Geometry: final body of the model. Coordinates: model frame, mm. A direction names the side the tool comes from. Coordinates: 2 decimals unless noted, no trailing zeros. Order: outer loops, then holes, each group sorted by start corner. A loop starts at its lowest first (then second) coordinate and runs counter-clockwise, first axis right, second up. Notation, with made-up numbers: (31.25, -38.75) -> (37.25, -38.75) arc R27 cw to (37.25, -5.75) -> close; hole circle Ø8 at (81, -34). An arc over 180 degrees is marked (long way). Answer in a Markdown table with one row per item. Add a question column.
1) Section query D-D on y = 61.5. Return the cut outline in (x, z), then the cut area to 3 significant figures.
2) Section query C-C on x = -33.5. Return the cut outline in (y, z), then the cut area to 3 significant figures.
3) Section query B-B on z = 143. Return the cut outline in (x, y), then the cut area to 3 significant figures.
4) Section query A-A on y = 35. Return the cut outline in (x, z).
5) Pull-direction query (Y, two-part tool) for faces 1 (the face through (-32, 85, 78)), 2 (the face through (10.809, 67.931, 77.302)), 3 (the face through (-31, -15, 78)); classes: +Y half, -Y half, draft (parallel to the pull), parting line (faces both ways), or undercut.
6) Contact query for flat-ended pins moving along their axis: P1, Ø8, axis at y = 0, z = 80, coming from the -X side; P2, Ø4, axis at x = -110.5, z = 147, coming from the +Y side; P3, Ø12, axis at x = -30.05, y = 35, coming from the -Z side; P4, Ø1, axis at y = 14.5, z = 31, coming from the -X side. Output: stop coordinate, or through.
7) Set-up query: faces 4 (the face through (10.809, -2.069, 77.302)), 5 (the face through (-55, 36, -34.286)). Return all of +Z, -Z, +X, -X, +Y, -Y with unobstructed straight access to the full face (end or side cutting, diameter ignored); none if empty.
8) Ray query, line 1 (Y direction, x = 4.5, z = 80); line 2 (Z direction, x = 17, y = 0); line 3 (X direction, y = 33, z = 143.5). Return the intervals inside material, ascending. Write a range as from..to.
```python
from build123d import *

# Parameters (mm, degrees)
BOSS_EXTRUDE1_DEPTH    = 160
SCALE1_SCALE           = 1.428571429
F_20_0MM_DOWEL_HOLE1_D = 20
M8_TAPPED_HOLE1_D      = 6.8
M8_TAPPED_HOLE1_DEPTH  = 22.25
M8_TAPPED_HOLE1_TIP    = 2.042926105


with BuildPart() as part:
    # Sketch1 → Boss-Extrude1 (new body)
    with BuildSketch(Plane.XY):
        with BuildLine():
            Line((0, 0), (-75, 0))
            ThreePointArc((-75, 0), (-110, 35), (-75, 70))
            Line((-75, 70), (0, 70))
            Line((0, 70), (0, 0))
        make_face()
    extrude(amount=BOSS_EXTRUDE1_DEPTH)


with BuildPart() as part_1:
    # Scale1: scaled about (-51.542183312, 35, 80)
    add(part.part.scale(SCALE1_SCALE).moved(Location((22.089507134, -15, -34.285714286))))

    # Ø20.0mm Dowel Hole1 (through all)
    with Locations(Plane(origin=(-30.053350009, 35, -34.285714286), x_dir=(-1, 0, 0), z_dir=(0, 0, -1))):
        with Locations((0, 0), (55, 0)):
            Hole(F_20_0MM_DOWEL_HOLE1_D / 2)

    # M8 Tapped Hole1
    with Locations(Plane(origin=(22.089507134, 0, 0), x_dir=(0, 0, -1), z_dir=(1, 0, 0))):
        with Locations((-80, 70), (-80, 0)):
            Hole(M8_TAPPED_HOLE1_D / 2, depth=M8_TAPPED_HOLE1_DEPTH)
            with Locations((0, 0, -(M8_TAPPED_HOLE1_DEPTH + M8_TAPPED_HOLE1_TIP / 2))):  # 118° drill point
                Cone(0, M8_TAPPED_HOLE1_D / 2, M8_TAPPED_HOLE1_TIP, mode=Mode.SUBTRACT)


solid = part_1.part
```
Result:
| question | item | result |
|---|---|---|
| 1 | outline | (-127.45, -34.29) -> (22.09, -34.29) -> (22.09, 194.29) -> (-127.45, 194.29) -> close |
| 1 | area | 34,200 mm2 |
| 2 | outline | (-15, -34.29) -> (25.61, -34.29) -> (25.61, 194.29) -> (-15, 194.29) -> close; (44.39, -34.29) -> (85, -34.29) -> (85, 194.29) -> (44.39, 194.29) -> close |
| 2 | area | 18,600 mm2 |
| 3 | outline | (-85.05, -15) -> (22.09, -15) -> (22.09, 85) -> (-85.05, 85) arc R50 ccw to start; hole circle Ø20 at (-85.05, 35); hole circle Ø20 at (-30.05, 35) |
| 3 | area | 14,000 mm2 |
| 4 | outline | (-135.05, -34.29) -> (-95.05, -34.29) -> (-95.05, 194.29) -> (-135.05, 194.29) -> close; (-75.05, -34.29) -> (-40.05, -34.29) -> (-40.05, 194.29) -> (-75.05, 194.29) -> close; (-20.05, -34.29) -> (22.09, -34.29) -> (22.09, 194.29) -> (-20.05, 194.29) -> close |
| 5 | face 1 | +Y half |
| 5 | face 2 | undercut |
| 5 | face 3 | -Y half |
| 6 | P1 | x = -124.28 |
| 6 | P2 | y = 79.16 |
| 6 | P3 | through |
| 6 | P4 | x = -130.88 |
| 7 | face 4 | +X |
| 7 | face 5 | -Z, +X, -X, +Y, -Y |
| 8 | line 1 | -15..-3.4, 3.4..66.6, 73.4..85 |
| 8 | line 2 | -34.29..76.6, 83.4..194.29 |
| 8 | line 3 | -135.01..-94.85, -75.26..-39.85, -20.26..22.09 |
